from build123d import *

# Parameters (mm, degrees)
SKETCH_1_R      = 4
EXTRUDE_1_DEPTH = 30
EXTRUDE_2_DEPTH = 2.5


with BuildPart() as part:
    # Эскиз1 → Бобышка-Вытянуть1 (new body)
    with BuildSketch(Plane(origin=(0, 0, 0), x_dir=(1, 0, 0), z_dir=(0, 1, 0))):
        with Locations(Location((0, 0, 0), (0, 0, 270))):
            Circle(SKETCH_1_R)
    extrude(amount=EXTRUDE_1_DEPTH)

    # Эскиз2 → Бобышка-Вытянуть2 (add)
    with BuildSketch(Plane(origin=(0, 30, 0), x_dir=(1, 0, 0), z_dir=(0, 1, 0))):
        with BuildLine():
            Line((30, 4), (30, 56))
            Line((30, 56), (34, 56))
            Line((34, 56), (34, -4))
            Line((34, -4), (11.842719282, -4))
            ThreePointArc((11.842719282, -4), (0, -12.5), (-11.842719282, -4))
            Line((-11.842719282, -4), (-30, -4))
            Line((-30, -4), (-30, -56))
            Line((-30, -56), (-34, -56))
            Line((-34, -56), (-34, 4))
            Line((-34, 4), (-11.842719282, 4))
            ThreePointArc((-11.842719282, 4), (0, 12.5), (11.842719282, 4))
            Line((11.842719282, 4), (30, 4))
        make_face()
    extrude(amount=EXTRUDE_2_DEPTH)


solid = part.part
Work out the finished part from the listing and answer in its coordinate system (mm). A direction names the side the tool comes from. Round coordinates to 2 decimals unless told otherwise and drop trailing zeros. Write each loop counter-clockwise with the first axis right and the second up, starting at its lowest first coordinate (ties: lowest second). Pieces come first, ordered by that corner, then holes. Notation, with made-up numbers: (86.25, 77) - (131.25, 77) arc R18 cw to (131.25, 100) - close; hole circle Ø8 at (6, 87.25). An arc over 180 degrees is marked (long way). Answer in a Markdown table with one row per item. Add a question column.
1. A cutting plane is placed at D-D, the plane x = -16.5. Determine the outline of the cut face in (y, z), and give its area (3 significant figures).
2. Given pin 1 (3 mm diameter, centred on x = 23, y = 31, fed in from -Z); pin 2 (20.5 mm diameter, centred on x = -6, z = -20, fed in from -Y); pin 3 (1.2 mm diameter, centred on y = 31.5, z = -18.5, fed in from -X), each flat-ended and moving along its own axis, determine where each tip first touches the part or whether it passes through.
3. A cutting plane is placed at C-C, the plane y = 10. Determine the outline of the cut face in (x, z).
4. The mould has two halves that part along X. Classify faces 4 (the cylindrical face through (-3.905, 14.79, -0.867)), 5 (the flat face through (32, 31, -56)), 6 (the cylindrical face through (-0.2, 31.2, -12.5)): +X half, -X half, draft (parallel to the pull), parting line (faces both ways), or undercut.
5. A cutting plane is placed at A-A, the plane x = 0. Determine the outline of the cut face in (y, z), and give its area (4 significant figures).
6. A cutting plane is placed at B-B, the plane z = 0. Determine the outline of the cut face in (x, y), and give its area (3 significant figures).
7. For faces 1 (the flat face through (-23, 31, -4)), 2 (the flat face through (-30, 31, 30)), 3 (the flat face through (23, 31, 4)), determine the directions among +Z, -Z, +X, -X, +Y, -Y from which every point of the face is accessible in a straight line to the end or side of a thin tool.
8. Find the intervals of material crossed by line 1 along Y through (x, z) = (-17, 2.5); line 2 along Z through (x, y) = (-3, 14.5); line 3 along Z through (x, y) = (2, 9), in increasing order. Write a range as from..to.
Worked out:
| question | item | result |
|---|---|---|
| 1 | outline | (30, -4) - (32.5, -4) - (32.5, 4) - (30, 4) - close |
| 1 | area | 20.0 mm^2 |
| 2 | pin 1 | z = -4 |
| 2 | pin 2 | y = 30 |
| 2 | pin 3 | x = 30 |
| 3 | outline | circle Ø8 at (0, 0) |
| 4 | face 4 | parting line |
| 4 | face 5 | draft |
| 4 | face 6 | undercut |
| 5 | outline | (0, -4) - (30, -4) - (30, -12.5) - (32.5, -12.5) - (32.5, 12.5) - (30, 12.5) - (30, 4) - (0, 4) - close |
| 5 | area | 302.5 mm^2 |
| 6 | outline | (-34, 30) - (-4, 30) - (-4, 0) - (4, 0) - (4, 30) - (34, 30) - (34, 32.5) - (-34, 32.5) - close |
| 6 | area | 410 mm^2 |
| 7 | face 1 | -Z, -X, +Y, -Y |
| 7 | face 2 | +Z, +Y, -Y |
| 7 | face 3 | +Z, +X, +Y, -Y |
| 8 | line 1 | 30..32.5 |
| 8 | line 2 | -2.65..2.65 |
| 8 | line 3 | -3.46..3.46 |
